Source: CAD feature listing. Evaluate the final solid. Frame: model axes, mm. Face numbers are marked on the shaded views. A direction names the side the tool comes from. Give positions to 0.01 mm unless a question says otherwise; leave off trailing zeros. Order: outer loops, then holes, each group sorted by start corner. A loop starts at its lowest first (then second) coordinate and runs counter-clockwise, first axis right, second up. Notation, with made-up numbers: (46.5, -17.75) -> (68.5, -17.75) arc R28 cw to (68.5, 7.25) -> close; hole circle Ø1 at (26.5, -7). An arc over 180 degrees is marked (long way). Answer in a Markdown table with one row per item.
Autodesk Fusion 360 part; units mm, degrees
sketch "Esboço1" plane through (0, 0, 0) normal (0, 1, 0) x (1, 0, 0)
  line L0 (0, 0) -> (56, 0)
  line L1 (56, -56) -> (0, -56)
  line L2 (0, -56) -> (0, 0)
  line L3 (0, -28) -> (45.1892, -28)
  arc A0 (56, -8.4245) -> (56, -34.4121) centre (56.4, -21.4183) ccw
  line L4 (56, 0) -> (56, -8.4245)
  line L5 (56, -34.4121) -> (56, -56)
  circle A1 centre (24.93, -7) radius 2.65
  circle A2 centre (33.9, -49) radius 2.65
  dimension "d1" = 56
  dimension "d2" = 56
  dimension "d3" = 26
  dimension "d5" = 5.3
  dimension "d6" = 24.93
  dimension "d7" = 21
  dimension "d8" = 5.3
  dimension "d9" = 21
  dimension "d10" = 33.9
  dimension "d47" = 56.4
extrude "Extrusão1" add sketch "Esboço1" along normal blind 3
sketch "Esboço2" plane through (0, 3, 0) normal (0, 1, 0) x (-1, 0, 0)
  circle A0 centre (-24.93, 7) radius 2.65
  circle A1 centre (-33.9, 49) radius 2.65
  arc A2 (-56, 8.4245) -> (-56, 34.4121) centre (-56.4, 21.4183) ccw
  line L0 (-56, 8.4245) -> (-56, 0)
  line L1 (-56, 0) -> (0, 0)
  line L2 (0, 0) -> (0, 56)
  line L3 (0, 56) -> (-56, 56)
  line L4 (-56, 56) -> (-56, 34.4121)
  line L5 (0, 0) -> (-3, 0)
  line L6 (-3, 0) -> (-3, 56)
  line L7 (-3, 56) -> (0, 56)
  line L8 (0, 56) -> (0, 0)
extrude "Extrusão2" add sketch "Esboço2" along normal blind 53 contours L1 L2 L3 L5 L6 L7 L8
sketch "Esboço3" plane through (0, 0, 0) normal (-1, 0, 0) x (0, 0, 1)
  line L0 (0, 0) -> (56, 0)
  line L1 (56, 0) -> (56, 56)
  line L2 (56, 56) -> (0, 56)
  line L3 (0, 56) -> (0, 0)
  circle A0 centre (28, 30) radius 13
  circle A1 centre (28, 14) radius 1.6
  circle A2 centre (14.1436, 38) radius 1.6
  circle A3 centre (41.8564, 38) radius 1.6
  dimension "d15" = 26
  dimension "d16" = 30
  dimension "d19" = 3.2
  dimension "d20" = 16
  dimension "d21" = 8
  dimension "d22" = 13.8564
extrude "Extrusão3" cut sketch "Esboço3" against normal blind 6.5 contours A0 | A1 | A2 | A3
sketch "Esboço6" plane through (3, 0, 0) normal (1, 0, 0) x (0, 0, -1)
  circle A0 centre (-41.8564, 38) radius 1.6
  circle A1 centre (-28, 14) radius 1.6
  circle A2 centre (-14.1436, 38) radius 1.6
  circle A3 centre (-28, 30) radius 13
  line L0 (-56, 3) -> (0, 3)
  line L1 (0, 3) -> (0, 56)
  line L2 (0, 56) -> (-56, 56)
  line L3 (-56, 56) -> (-56, 3)
  line L4 (-56, 56) -> (0, 56)
  line L5 (0, 56) -> (0, 53)
  line L6 (0, 53) -> (-56, 53)
  line L7 (-56, 53) -> (-56, 56)
  dimension "d48" = 3
extrude "Extrusão6" add sketch "Esboço6" along normal blind 53 contours L1 L2 L3 L4 L5 L6 L7
sketch "Esboço7" plane through (0, 53, 0) normal (0, -1, 0) x (1, 0, 0)
  line L0 (3, 56) -> (3, 0)
  line L1 (3, 0) -> (56, 0)
  line L2 (56, 0) -> (56, 56)
  line L3 (56, 56) -> (3, 56)
  line L4 (56, 0) -> (53, 0)
  line L5 (53, 0) -> (53, 56)
  line L6 (53, 56) -> (56, 56)
  line L7 (56, 56) -> (56, 0)
  dimension "d51" = 3
extrude "Extrusão7" add sketch "Esboço7" along normal blind 50 contours L1 L2 L3 L4 L5 L6 L7
sketch "Esboço8" plane through (0, 0, 0) normal (0, -1, 0) x (1, 0, 0)
  circle A0 centre (33.9, 49) radius 2.65
  circle A1 centre (24.93, 7) radius 2.65
  arc A2 (56, 34.4121) -> (56, 8.4245) centre (56.4, 21.4183) ccw
  line L0 (56, 34.4121) -> (56, 56)
  line L1 (56, 56) -> (0, 56)
  line L2 (0, 56) -> (0, 0)
  line L3 (0, 0) -> (56, 0)
  line L4 (56, 0) -> (56, 8.4245)
  circle A3 centre (56.4, 21.4183) radius 13
extrude "Extrusão8" cut sketch "Esboço8" against normal blind 69 contours A2 A3
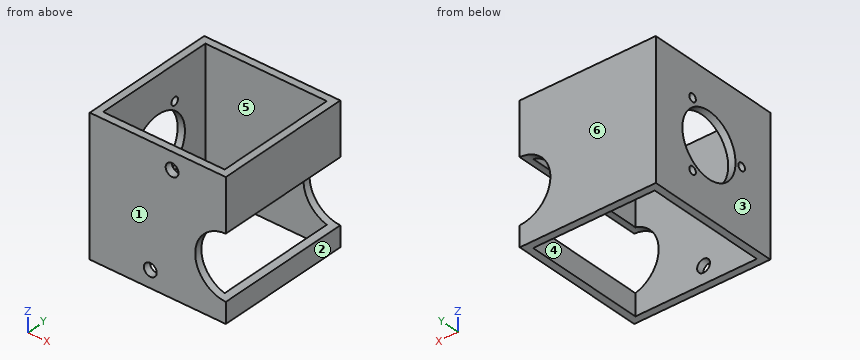
(1) Section query D-D (z = 7). Return the cut outline in (x, y).
A:
| item | result |
|---|---|
| outline | (0, 0) -> (22.28, 0) -> (22.28, 3) -> (3, 3) -> (3, 53) -> (53, 53) -> (53, 3) -> (27.58, 3) -> (27.58, 0) -> (56, 0) -> (56, 56) -> (0, 56) -> close |
(2) Access query for the marked faces 5 and 6. Directions: +Z, -Z, +X, -X, +Y, -Y. A direction counts if a zero-diameter tool reaches every point of the face in a straight line with its end or side. Return the directions, or none.
A:
| item | result |
|---|---|
| face 5 | +Z, -Z |
| face 6 | +Z, -Z, +X, -X, +Y |
(3) Section query B-B (x = 33.9). Return the cut outline in (y, z), plus the area to 3 significant figures.
A:
| item | result |
|---|---|
| outline | (0, 0) -> (3, 0) -> (3, 46.35) -> (0, 46.35) -> close; (0, 51.65) -> (3, 51.65) -> (3, 56) -> (0, 56) -> close; (53, 0) -> (56, 0) -> (56, 56) -> (53, 56) -> close |
| area | 320 mm^2 |
(4) Pull-direction query (X, two-part tool) for the marked faces 1, 2, 3 and 4; classes: +X half, -X half, draft (parallel to the pull), parting line (faces both ways), or undercut.
A:
| item | result |
|---|---|
| face 1 | draft |
| face 2 | +X half |
| face 3 | -X half |
| face 4 | undercut |
(5) Ray query, probe 1 along Y at (x, z) = (2.05, 28); probe 2 along Y at (x, z) = (16.5, 48). Return the intervals inside material, ascending.
A:
| item | result |
|---|---|
| probe 1 | y = 0 to 12.4, 15.6 to 17, 43 to 56 |
| probe 2 | y = 0 to 3, 53 to 56 |
(6) Section query A-A (y = 30). Return the cut outline in (x, z).
A:
| item | result |
|---|---|
| outline | (0, 0) -> (3, 0) -> (3, 15) -> (0, 15) -> close; (0, 41) -> (3, 41) -> (3, 56) -> (0, 56) -> close; (53, 0) -> (56, 0) -> (56, 8.42) arc R13 cw to (53, 8.87) -> close; (53, 33.97) arc R13 cw to (56, 34.41) -> (56, 56) -> (53, 56) -> close |
(7) Section query C-C (x = 40.5). Return the cut outline in (y, z), plus the area to 3 significant figures.
A:
| item | result |
|---|---|
| outline | (0, 0) -> (3, 0) -> (3, 56) -> (0, 56) -> close; (53, 0) -> (56, 0) -> (56, 56) -> (53, 56) -> close |
| area | 336 mm^2 |
(8) First-contact query: pin 1 Ø1.9 at (y, z) = (38, 14.14) entering from -X; pin 2 Ø3 at (y, z) = (38, 41.86) entering from -X; pin 3 Ø4 at (y, z) = (19, 31.5) entering from +X; pin 4 Ø5 at (x, z) = (33.9, 49) entering from -Y. Flat tips, straight axial feed; report the tip coordinate or a pass-through.
A:
| item | result |
|---|---|
| pin 1 | passes through |
| pin 2 | stops at x = 53 |
| pin 3 | stops at x = 3 |
| pin 4 | stops at y = 53 |
